Source: CAD feature listing. Evaluate the final solid. Frame: model axes, mm. A direction names the side the tool comes from. Coordinates: 2 decimals unless noted, no trailing zeros. Write each loop counter-clockwise with the first axis right and the second up, starting at its lowest first coordinate (ties: lowest second). Pieces come first, ordered by that corner, then holes. Notation, with made-up numbers: (6.5, -22.5) - (23.5, -22.5) arc R28 ccw to (23.5, 9.5) - close; hole circle Ø6 at (59, 20). An arc over 180 degrees is marked (long way). One line per question, with ' | ' between items. Start each with the question number.
Q1. Access query for faces 1 (the face through (10.422, 144.556, -12.808)), 2 (the face through (-20, 146, 3.5)), 3 (the face through (-3.5, 146, 20)), 4 (the face through (20, 146, -3.5)), 5 (the face through (-5.26, -4.44, 18.45)). Directions: +Z, -Z, +X, -X, +Y, -Y. A direction counts if a zero-diameter tool reaches every point of the face in a straight line with its end or side. Return the directions, or none.
Q2. Cut plane A-A, the plane y = 126. Return loops of the section in (x, z), plus the area to 3 significant figures.
Q3. Line query: line 1 (Y direction, x = 2.5, z = -7); line 2 (Y direction, x = -9, z = 18.5); line 3 (Z direction, x = 17, y = 138). Output: solid intervals per line, ascending.
Q4. Contact query for flat-ended pins moving along their axis: P1, Ø1.5, axis at x = 16.5, y = 79.5, coming from the +Z side; P2, Ø12, axis at x = 11.5, y = 61, coming from the -Z side; P3, Ø1, axis at x = 10.5, z = -14.5, coming from the -Y side. Output: stop coordinate, or through.
Q5. Cut plane C-C, the plane y = 159.5. Return loops of the section in (x, z).
Q6. Cut plane B-B, the plane x = -8.5. Return loops of the section in (y, z).
Q7. Draft query along X for faces 6 (the face through (6.536, -4.563, 15.46)), 7 (the face through (0, -4, 9.376)), 8 (the face through (12, 140.5, 12)), 9 (the face through (-7.91, 149.486, -10.316)). Return one class per face: +X half, -X half, draft (parallel to the pull), parting line (faces both ways), or undercut.
```python
from build123d import *

# Parameters (mm, degrees)
SKETCH1_R           = 22.5
BOSS_EXTRUDE1_DEPTH = 78
SKETCH2_R           = 22.5
BOSS_EXTRUDE2_DEPTH = 70.5
SKETCH3_R           = 13
BOSS_EXTRUDE3_DEPTH = 2
BOSS_EXTRUDE4_DEPTH = 20
SKETCH5_R           = 5
BOSS_EXTRUDE5_DEPTH = 7
SKETCH6_R           = 2
CUT_EXTRUDE1_DEPTH  = 8
CUT_EXTRUDE2_START  = -5
CUT_EXTRUDE2_DEPTH  = 5
SKETCH8_R           = 2
CUT_EXTRUDE3_DEPTH  = 8
BOSS_EXTRUDE6_DEPTH = 9
SKETCH10_R          = 5.5
BOSS_EXTRUDE7_DEPTH = 5
FILLET1_R           = 3
FILLET2_R           = 2
SKETCH11_R          = 5.5
BOSS_EXTRUDE8_DEPTH = 1
FILLET3_R           = 1


with BuildPart() as part:
    # Sketch1 → Boss-Extrude1 (new body)
    with BuildSketch(Plane(origin=(0, 0, 0), x_dir=(1, 0, 0), z_dir=(0, 1, 0))):
        with Locations(Location((0, 0, 0), (0, 0, 270))):
            Circle(SKETCH1_R)
    extrude(amount=BOSS_EXTRUDE1_DEPTH)

    # Sketch2 → Boss-Extrude2 (add)
    with BuildSketch(Plane(origin=(0, 78, 0), x_dir=(1, 0, 0), z_dir=(0, 1, 0))):
        with Locations(Location((0, 0, 0), (0, 0, 270))):
            Circle(SKETCH2_R)
    extrude(amount=BOSS_EXTRUDE2_DEPTH)

    # Sketch3 → Boss-Extrude3 (add)
    with BuildSketch(Plane(origin=(0, 148.5, 0), x_dir=(1, 0, 0), z_dir=(0, 1, 0))):
        with Locations(Location((0, 0, 0), (0, 0, 270))):
            Circle(SKETCH3_R)
    extrude(amount=BOSS_EXTRUDE3_DEPTH)

    # Sketch4 → Boss-Extrude4 (add)
    with BuildSketch(Plane(origin=(0, 150.5, 0), x_dir=(1, 0, 0), z_dir=(0, 1, 0))):
        with BuildLine():
            ThreePointArc((-4, 3), (-4.472135955, -2.236067977), (0, -5))
            Line((0, -5), (0, 3))
            Line((0, 3), (-4, 3))
        make_face()
        with BuildLine():
            Line((0, 3), (0, -5))
            ThreePointArc((0, -5), (3.535533906, -3.535533906), (5, 0))
            ThreePointArc((5, 0), (4.74341649, 1.58113883), (4, 3))
            Line((4, 3), (0, 3))
        make_face()
    extrude(amount=BOSS_EXTRUDE4_DEPTH)

    # Sketch5 → Boss-Extrude5 (add)
    with BuildSketch(Plane(origin=(0, 150.5, 0), x_dir=(1, 0, 0), z_dir=(0, 1, 0))):
        with Locations(Location((0, 0, 0), (0, 0, 143.130102354))):
            Circle(SKETCH5_R)
    extrude(amount=BOSS_EXTRUDE5_DEPTH)

    # Sketch6 → Cut-Extrude1 (cut)
    with BuildSketch(Plane(origin=(0, 148.5, 0), x_dir=(1, 0, 0), z_dir=(0, 1, 0))):
        with Locations(Location((-12.374368671, 12.374368671, 0), (0, 0, 270))):
            Circle(SKETCH6_R)
        with Locations(Location((12.374368671, 12.374368671, 0), (0, 0, 270))):
            Circle(SKETCH6_R)
        with Locations(Location((12.374368671, -12.374368671, 0), (0, 0, 270))):
            Circle(SKETCH6_R)
        with Locations(Location((-12.374368671, -12.374368671, 0), (0, 0, 270))):
            Circle(SKETCH6_R)
    extrude(amount=-CUT_EXTRUDE1_DEPTH, mode=Mode.SUBTRACT)

    # Sketch7 → Cut-Extrude2 (cut)
    with BuildSketch(Plane(origin=(0, 148.5, 0), x_dir=(1, 0, 0), z_dir=(0, 1, 0)).offset(CUT_EXTRUDE2_START)):
        with BuildLine():
            ThreePointArc((22.5, 0), (22.431423187, 1.755350058), (22.226110771, 3.5))
            Line((22.226110771, 3.5), (17.5, 3.5))
            ThreePointArc((17.5, 3.5), (19.974873734, 2.474873734), (21, 0))
            ThreePointArc((21, 0), (19.974873734, -2.474873734), (17.5, -3.5))
            Line((17.5, -3.5), (22.226110771, -3.5))
            ThreePointArc((22.226110771, -3.5), (22.431423187, -1.755350058), (22.5, 0))
        make_face()
        with BuildLine():
            ThreePointArc((21, 0), (19.974873734, 2.474873734), (17.5, 3.5))
            Line((17.5, 3.5), (17.5, -3.5))
            ThreePointArc((17.5, -3.5), (19.974873734, -2.474873734), (21, 0))
        make_face()
        with BuildLine():
            Line((17.5, -3.5), (17.5, 3.5))
            ThreePointArc((17.5, 3.5), (14, 0), (17.5, -3.5))
        make_face()
        with BuildLine():
            ThreePointArc((3.5, 22.226110771), (1.755350006, 22.431423191), (-1.05e-07, 22.5))
            ThreePointArc((-1.05e-07, 22.5), (-1.755350111, 22.431423182), (-3.5, 22.226110771))
            Line((-3.5, 22.226110771), (-3.5, 17.5))
            ThreePointArc((-3.5, 17.5), (0, 21), (3.5, 17.5))
            Line((3.5, 17.5), (3.5, 22.226110771))
        make_face()
        with BuildLine():
            ThreePointArc((3.5, 17.5), (0, 21), (-3.5, 17.5))
            Line((-3.5, 17.5), (3.5, 17.5))
        make_face()
        with BuildLine():
            Line((3.5, 17.5), (-3.5, 17.5))
            ThreePointArc((-3.5, 17.5), (0, 14), (3.5, 17.5))
        make_face()
        with BuildLine():
            ThreePointArc((-14, 0), (-15.025126266, 2.474873734), (-17.5, 3.5))
            Line((-17.5, 3.5), (-17.5, -3.5))
            ThreePointArc((-17.5, -3.5), (-15.025126266, -2.474873734), (-14, 0))
        make_face()
        with BuildLine():
            Line((-17.5, -3.5), (-17.5, 3.5))
            ThreePointArc((-17.5, 3.5), (-21, 0), (-17.5, -3.5))
        make_face()
        with BuildLine():
            Line((-17.5, 3.5), (-22.226110771, 3.5))
            ThreePointArc((-22.226110771, 3.5), (-22.431423191, 1.755350006), (-22.5, -1.05e-07))
            ThreePointArc((-22.5, -1.05e-07), (-22.431423182, -1.755350111), (-22.226110771, -3.5))
            Line((-22.226110771, -3.5), (-17.5, -3.5))
            ThreePointArc((-17.5, -3.5), (-21, 0), (-17.5, 3.5))
        make_face()
        with BuildLine():
            ThreePointArc((3.5, -17.5), (0, -14), (-3.5, -17.5))
            Line((-3.5, -17.5), (3.5, -17.5))
        make_face()
        with BuildLine():
            Line((3.5, -17.5), (-3.5, -17.5))
            ThreePointArc((-3.5, -17.5), (0, -21), (3.5, -17.5))
        make_face()
        with BuildLine():
            Line((-3.5, -17.5), (-3.5, -22.226110771))
            ThreePointArc((-3.5, -22.226110771), (-1.755350006, -22.431423191), (1.05e-07, -22.5))
            ThreePointArc((1.05e-07, -22.5), (1.755350111, -22.431423182), (3.5, -22.226110771))
            Line((3.5, -22.226110771), (3.5, -17.5))
            ThreePointArc((3.5, -17.5), (0, -21), (-3.5, -17.5))
        make_face()
    extrude(amount=CUT_EXTRUDE2_DEPTH, mode=Mode.SUBTRACT)

    # Sketch8 → Cut-Extrude3 (cut)
    with BuildSketch(Plane(origin=(0, 143.5, 0), x_dir=(1, 0, 0), z_dir=(0, 1, 0))):
        with Locations(Location((0, 17.5, 0), (0, 0, 270))):
            Circle(SKETCH8_R)
        with Locations(Location((17.5, 0, 0), (0, 0, 270))):
            Circle(SKETCH8_R)
        with Locations(Location((0, -17.5, 0), (0, 0, 270))):
            Circle(SKETCH8_R)
        with Locations(Location((-17.5, 0, 0), (0, 0, 270))):
            Circle(SKETCH8_R)
    extrude(amount=-CUT_EXTRUDE3_DEPTH, mode=Mode.SUBTRACT)

    # Sketch9 → Boss-Extrude6 (add)
    with BuildSketch(Plane.XZ):
        Polygon((-3.5, 21.5), (3.5, 21.5), (7, 15.437822174), (3.5, 9.375644347), (-3.5, 9.375644347), (-7, 15.437822174), align=None)
    extrude(amount=BOSS_EXTRUDE6_DEPTH)

    # Sketch10 → Boss-Extrude7 (add)
    with BuildSketch(Plane.XZ.offset(9)):
        with Locations(Location((0, 15.437822174, 0), (0, 0, 270))):
            Circle(SKETCH10_R)
    extrude(amount=BOSS_EXTRUDE7_DEPTH)

    # Fillet1
    fillet1_edges = [part.edges().sort_by_distance(p)[0] for p in [
        (-3.5, -4.5, 21.5),
        (-7, -4.5, 15.437822174),
        (-3.5, -4.5, 9.375644347),
        (3.5, -4.5, 9.375644347),
        (7, -4.5, 15.437822174),
        (3.5, -4.5, 21.5),
    ]]
    fillet(fillet1_edges, radius=FILLET1_R)

    # Fillet2
    fillet2_edges = [part.edges().sort_by_distance(p)[0] for p in [
        (0, -14, 20.937822174),
    ]]
    fillet(fillet2_edges, radius=FILLET2_R)

    # Sketch11 → Boss-Extrude8 (add)
    with BuildSketch(Plane.XZ):
        with Locations(Location((0, 0, 0), (0, 0, 90))):
            Circle(SKETCH11_R)
    extrude(amount=BOSS_EXTRUDE8_DEPTH)

    # Fillet3
    fillet3_edges = [part.edges().sort_by_distance(p)[0] for p in [
        (0, -1, -5.5),
    ]]
    fillet(fillet3_edges, radius=FILLET3_R - 0.0001)  # a hair under: the kernel refuses the full size


solid = part.part
```
Reply:
1) face 1: +Y | face 2: -X, +Y | face 3: +Z, +Y | face 4: +X, +Y | face 5: +Z, -X, -Y
2) outline: circle Ø45 at (0, 0) | area: 1,590 mm^2
3) line 1: y = 0 to 150.5 | line 2: y = 0 to 148.5 | line 3: z = -14.74 to -1.94, 1.94 to 14.74
4) P1: stops at z = 16.07 | P2: stops at z = -21.82 | P3: stops at y = 0
5) outline: (-4, -3) - (4, -3) arc R5 ccw (long way) to start
6) outline: (0, -20.83) - (148.5, -20.83) - (148.5, -9.84) - (150.5, -9.84) - (150.5, 9.84) - (148.5, 9.84) - (148.5, 20.83) - (0, 20.83) - close
7) face 6: +X half | face 7: draft | face 8: undercut | face 9: parting line
